from build123d import *

# Parameters (mm, degrees)
F0_R     = 0.85
F1_DEPTH = 3.5


with BuildPart() as f1:
    # F0 (on Top) → F1 (new body)
    with BuildSketch(Plane.XY):
        with BuildLine():
            Line((-6.363693, -0.75), (6.363693, -0.75))
            ThreePointArc((6.363693, -0.75), (9.449299, -1.067488), (8.23095, 1.785122))
            Line((8.23095, 1.785122), (0, 2.85))
            Line((0, 2.85), (-8.23095, 1.785122))
            ThreePointArc((-8.23095, 1.785122), (-9.449299, -1.067488), (-6.363693, -0.75))
        make_face()
        with Locations((-8, 0)):
            Circle(F0_R, mode=Mode.SUBTRACT)
        with Locations((8, 0)):
            Circle(F0_R, mode=Mode.SUBTRACT)
    extrude(amount=F1_DEPTH)


solid = f1.part
Can you work these out from the model? Positions are in its coordinate system, mm. A direction names the side the tool comes from. Give positions to 0.01 mm unless a question says otherwise; leave off trailing zeros. Loops run counter-clockwise (first coordinate to the right, second up) from the corner with the lowest first, then second, coordinate; pieces in that order, holes last. Notation, with made-up numbers: (73, 61) -> (84, 61) arc R28 ccw to (84, 97) -> close; hole circle Ø5 at (27, 7.25). An arc over 180 degrees is marked (long way). Write item = value, one per line.
1) Will these pins go through, and if not, where does the flat tip stop? pin 1 (1 mm diameter, centred on x = -4.5, z = 2.5, fed in from -Y); pin 2 (2 mm diameter, centred on x = -6.5, z = 2, fed in from -Y).
Check result:
pin_1 = -0.75
pin_2 = -1.73
2) For faces 1 (the flat face through (0, -0.75, 2)), 2 (the cylindrical face through (9.418, -1.109, 1.726)), which set-ups out of +Z, -Z, +X, -X, +Y, -Y let a thin tool reach every point of the face, with its end or its side?
Check result:
face_1 = +Z, -Z, -Y
face_2 = +Z, -Z
3) Suppose I cut it at D-D on y = -1.05. Write out the boundary of the cut face in (x, z), then the cut area to 3 significant figures.
Check result:
outline = (-9.46, 0) -> (-6.54, 0) -> (-6.54, 3.5) -> (-9.46, 3.5) -> close; (6.54, 0) -> (9.46, 0) -> (9.46, 3.5) -> (6.54, 3.5) -> close
area = 20.5 mm2
4) Suppose I cut it at B-B on y = 0. Write out the boundary of the cut face in (x, z), then the cut area to 3 significant figures.
Check result:
outline = (-9.8, 0) -> (-8.85, 0) -> (-8.85, 3.5) -> (-9.8, 3.5) -> close; (-7.15, 0) -> (7.15, 0) -> (7.15, 3.5) -> (-7.15, 3.5) -> close; (8.85, 0) -> (9.8, 0) -> (9.8, 3.5) -> (8.85, 3.5) -> close
area = 56.7 mm2
5) I need wall thicknesses on L1, parallel to X at y = -0.65, z = 0.9; L2, parallel to Y at x = -8, z = 2.6 (3 decimals); L3, parallel to Y at x = -6, z = 1.7. Which ranges of each line are inside material? Lowest first, please. Write a range as from..to.
Check result:
L1 = -9.68..-8.55, -7.45..7.45, 8.55..9.68
L2 = -1.8..-0.85, 0.85..1.815
L3 = -0.75..2.07
6) Thinking about a two-plate mould opening in X: for faces 3 (the flat face through (-4.058, 2.325, 1.726)), 4 (the cylindrical face through (-7.215, -0.326, 1.726)), 5 (the cylindrical face through (-9.48, -1.025, 1.726)), 6 (the flat face through (0, 1, 3.5)), which applies, released by +X, released by -X, zero draft, split by the parting line, or undercut?
Check result:
face_3 = released by -X
face_4 = undercut
face_5 = undercut
face_6 = zero draft
7) Suppose I cut it at C-C on x = 8. Write out the boundary of the cut face in (y, z) (3 decimals), then the cut area to 3 significant figures.
Check result:
outline = (-1.8, 0) -> (-0.85, 0) -> (-0.85, 3.5) -> (-1.8, 3.5) -> close; (0.85, 0) -> (1.815, 0) -> (1.815, 3.5) -> (0.85, 3.5) -> close
area = 6.70 mm2
8) Suppose I cut it at A-A on z = 1.3. Write out the boundary of the cut face in (x, y).
Check result:
outline = (-8.23, 1.79) arc R1.8 ccw (long way) to (-6.36, -0.75) -> (6.36, -0.75) arc R1.8 ccw (long way) to (8.23, 1.79) -> (0, 2.85) -> close; hole circle Ø1.7 at (-8, 0); hole circle Ø1.7 at (8, 0)
